from build123d import *

# Parameters (mm, degrees)
SKETCH_2_W                       = 64.02174429
SKETCH_2_H                       = 9.248919907
CUT_EXTRUDE_1_DEPTH              = 49
HOLE_WIZARD_M4_2_D               = 3.3
HOLE_WIZARD_M4_2_DEPTH           = 5.5
HOLE_WIZARD_M4_2_TIP             = 0.991420021
HOLE_WIZARD_M6_2_D               = 5
HOLE_WIZARD_M6_2_DEPTH           = 5.5
HOLE_WIZARD_M6_2_TIP             = 1.502151548
HOLE_WIZARD_M4_3_D               = 3.3
HOLE_WIZARD_M4_3_DEPTH           = 13.4
HOLE_WIZARD_M4_3_TIP             = 0.991420021
HOLE_WIZARD_M4_3_ON_FACE_2_D     = 3.3
HOLE_WIZARD_M4_3_ON_FACE_2_DEPTH = 13.4
HOLE_WIZARD_M4_3_ON_FACE_2_TIP   = 0.991420021


with BuildPart() as part:
    # 草图1 → 旋转1 (revolve)
    with BuildSketch(Plane(origin=(0, 0, 0), x_dir=(1, 0, 0), z_dir=(0, 1, 0)), mode=Mode.PRIVATE) as revolve_1_sk:
        Polygon((25.4, 7.5), (25.4, -7.5), (15.875, -7.5), (15.875, -4), (16.975, -4), (16.975, 4), (15.875, 4), (15.875, 7.5), align=None)
    revolve(revolve_1_sk.sketch.rotate(Axis((0, 0, -31.9390681), (0, 0, 1)), 180), axis=Axis((0, 0, -31.9390681), (0, 0, 1)))  # turned: the seam where the file's is

    # 草图2 → 切除-拉伸1 (cut)
    with BuildSketch(Plane.XY.offset(7.5)):
        with Locations((-1.141100508, 29.124459954)):
            Rectangle(SKETCH_2_W, SKETCH_2_H)
        with Locations((-1.141100508, -29.124459954)):
            Rectangle(SKETCH_2_W, SKETCH_2_H)
    extrude(amount=-CUT_EXTRUDE_1_DEPTH, mode=Mode.SUBTRACT)

    # M4 螺纹孔2
    with Locations(Plane(origin=(0, 24.5, 0), x_dir=(1, 0, 0), z_dir=(0, 1, 0))):
        with Locations((0, 0)):
            Hole(HOLE_WIZARD_M4_2_D / 2, depth=HOLE_WIZARD_M4_2_DEPTH)
            with Locations((0, 0, -(HOLE_WIZARD_M4_2_DEPTH + HOLE_WIZARD_M4_2_TIP / 2))):  # 118° drill point
                Cone(0, HOLE_WIZARD_M4_2_D / 2, HOLE_WIZARD_M4_2_TIP, mode=Mode.SUBTRACT)

    # M6 螺纹孔2
    with Locations(Plane(origin=(0, -24.5, 0), x_dir=(-1, 0, 0), z_dir=(0, -1, 0))):
        with Locations((0, 0)):
            Hole(HOLE_WIZARD_M6_2_D / 2, depth=HOLE_WIZARD_M6_2_DEPTH)
            with Locations((0, 0, -(HOLE_WIZARD_M6_2_DEPTH + HOLE_WIZARD_M6_2_TIP / 2))):  # 118° drill point
                Cone(0, HOLE_WIZARD_M6_2_D / 2, HOLE_WIZARD_M6_2_TIP, mode=Mode.SUBTRACT)

    # M4 螺纹孔3
    with Locations(Plane(origin=(21.997045256, 12.7, 0), x_dir=(-0.5, 0.866025404, 0), z_dir=(0.866025404, 0.5, 0))):
        with Locations((0, 0)):
            Hole(HOLE_WIZARD_M4_3_D / 2, depth=HOLE_WIZARD_M4_3_DEPTH)
            with Locations((0, 0, -(HOLE_WIZARD_M4_3_DEPTH + HOLE_WIZARD_M4_3_TIP / 2))):  # 118° drill point
                Cone(0, HOLE_WIZARD_M4_3_D / 2, HOLE_WIZARD_M4_3_TIP, mode=Mode.SUBTRACT)

    # M4 螺纹孔3 on face 2
    with Locations(Plane(origin=(-21.997045256, 12.7, 0), x_dir=(-0.500000175, -0.866025303, 0), z_dir=(-0.866025303, 0.500000175, 0))):
        with Locations((0, 0)):
            Hole(HOLE_WIZARD_M4_3_ON_FACE_2_D / 2, depth=HOLE_WIZARD_M4_3_ON_FACE_2_DEPTH)
            with Locations((0, 0, -(HOLE_WIZARD_M4_3_ON_FACE_2_DEPTH + HOLE_WIZARD_M4_3_ON_FACE_2_TIP / 2))):  # 118° drill point
                Cone(0, HOLE_WIZARD_M4_3_ON_FACE_2_D / 2, HOLE_WIZARD_M4_3_ON_FACE_2_TIP, mode=Mode.SUBTRACT)


solid = part.part
For this review, take the finished solid that the model builds, in its own axes (mm). A direction names the side the tool comes from. Coordinates: 2 decimals unless noted, no trailing zeros. Order: outer loops, then holes, each group sorted by start corner. A loop starts at its lowest first (then second) coordinate and runs counter-clockwise, first axis right, second up. Notation, with made-up numbers: (77.5, 72) -> (94.5, 72) arc R23 cw to (94.5, 88) -> close; hole circle Ø2 at (86.25, 43.5). An arc over 180 degrees is marked (long way). Return JSON: item names as keys, results as strings.
1. We need section A-A on y = 0. Write out the cut boundary in (x, z) (3 decimals).
Answer block:
{"outline": "(-25.4, -7.5) -> (-15.875, -7.5) -> (-15.875, -4) -> (-16.975, -4) -> (-16.975, 4) -> (-15.875, 4) -> (-15.875, 7.5) -> (-25.4, 7.5) -> close; (15.875, -7.5) -> (25.4, -7.5) -> (25.4, 7.5) -> (15.875, 7.5) -> (15.875, 4) -> (16.975, 4) -> (16.975, -4) -> (15.875, -4) -> close"}
2. Machinability: for faces 4 (the flat face through (-3, -24.5, 0)), 5 (the flat face through (15, 6, 4)), 6 (the cylindrical face through (-0.54, -21.71, 2.44)), which of the approach directions +Z, -Z, +X, -X, +Y, -Y give a long, thin tool a straight path to every point of the face, cutting with its end or side? Answer none if there is none.
Answer block:
{"face 4": "+Z, -Z, +X, -X, -Y", "face 5": "none", "face 6": "-Y"}
3. We need section D-D on y = -20.5. Write out the cut boundary in (x, z), and give its area (3 significant figures).
Answer block:
{"outline": "(-15, -7.5) -> (15, -7.5) -> (15, 7.5) -> (-15, 7.5) -> close; hole circle Ø5 at (0, 0)", "area": "430 mm²"}
4. We need section C-C on y = 21. Write out the cut boundary in (x, z), and give its area (3 significant figures).
Answer block:
{"outline": "(-14.29, -7.5) -> (14.29, -7.5) -> (14.29, 7.5) -> (-14.29, 7.5) -> close; hole circle Ø3.3 at (0, 0)", "area": "420 mm²"}
5. For line 1 (Y direction, x = 0, z = -5.95) (3 decimals); line 2 (Z direction, x = 0, y = -22); line 3 (Y direction, x = -7.5, z = -3), list the stretches that pass through material, from the lowest coordinate up. Write a range as from..to.
Answer block:
{"line 1": "-24.5..-15.875, 15.875..24.5", "line 2": "-7.5..-2.5, 2.5..7.5", "line 3": "-24.27..-15.23, 15.23..24.27"}
6. For pin 1 Ø3 at (x, z) = (0, 0) entering from +Y; pin 2 Ø4 at (x, z) = (-15.5, -4.5) entering from +Y; pin 3 Ø17 at (x, y) = (4, -2) entering from -Z; pin 4 Ø4 at (x, z) = (-10, -2) entering from +Y, all flat-tipped, find the tip position at first contact; note any pin that passes through.
Answer block:
{"pin 1": "y = 18.91", "pin 2": "y = 21.52", "pin 3": "through", "pin 4": "y = 24.11"}
7. The part is to be moulded in two halves that separate along Y. For faces 1 (the cylindrical face through (-16.19, -5.1, -0.06)), 2 (the cylindrical face through (25.396, -0.464, 0.105)), 3 (the cylindrical face through (1.216, 21.712, -1.115)), say which applies: +Y half, -Y half, draft (parallel to the pull), parting line (faces both ways), or undercut.
Answer block:
{"face 1": "undercut", "face 2": "parting line", "face 3": "draft"}
8. We need section B-B on x = -4.5. Write out the cut boundary in (y, z), and give its area (3 significant figures).
Answer block:
{"outline": "(-24.5, -7.5) -> (-15.22, -7.5) -> (-15.22, -4) -> (-16.37, -4) -> (-16.37, 4) -> (-15.22, 4) -> (-15.22, 7.5) -> (-24.5, 7.5) -> close; (15.22, -7.5) -> (24.5, -7.5) -> (24.5, 7.5) -> (15.22, 7.5) -> (15.22, 4) -> (16.37, 4) -> (16.37, -4) -> (15.22, -4) -> close", "area": "260 mm²"}
